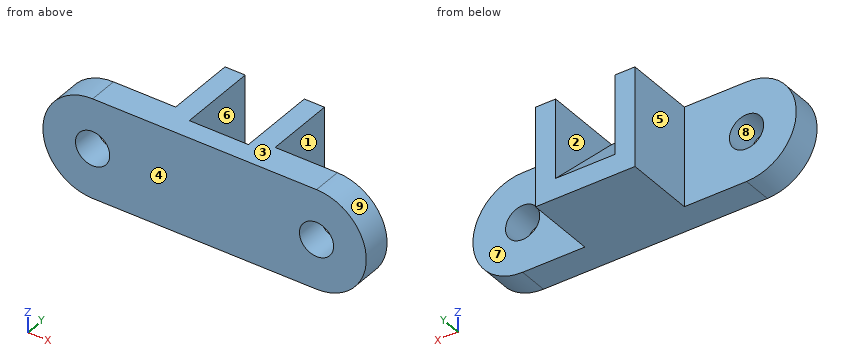
from build123d import *

# Parameters (mm, degrees)
SKETCH1_R           = 11
BOSS_EXTRUDE1_DEPTH = 19
SKETCH2_W           = 64
SKETCH2_H           = 64
BOSS_EXTRUDE2_DEPTH = 45
CUT_EXTRUDE2_START  = -13
CUT_EXTRUDE2_DEPTH  = 38


with BuildPart() as part:
    # Sketch1 → Boss-Extrude1 (new body)
    with BuildSketch(Plane(origin=(0, 0, 0), x_dir=(1, 0, 0), z_dir=(0, 1, 0))):
        with BuildLine():
            Line((-72, 32), (72, 32))
            ThreePointArc((72, 32), (104, 0), (72, -32))
            Line((72, -32), (-72, -32))
            ThreePointArc((-72, -32), (-104, 0), (-72, 32))
        make_face()
        with Locations(Location((-72, 0, 0), (0, 0, 270))):
            Circle(SKETCH1_R, mode=Mode.SUBTRACT)
        with Locations(Location((72, 0, 0), (0, 0, 270))):
            Circle(SKETCH1_R, mode=Mode.SUBTRACT)
    extrude(amount=BOSS_EXTRUDE1_DEPTH)

    # Sketch2 → Boss-Extrude2 (add)
    with BuildSketch(Plane(origin=(0, 19, 0), x_dir=(1, 0, 0), z_dir=(0, 1, 0))):
        Rectangle(SKETCH2_W, SKETCH2_H)
    extrude(amount=BOSS_EXTRUDE2_DEPTH)

    # Sketch4 → Cut-Extrude2 (cut)
    with BuildSketch(Plane.ZY.offset(32).offset(CUT_EXTRUDE2_START)):
        Polygon((32, 64), (-19, 64), (32, 13), align=None)
    extrude(amount=-CUT_EXTRUDE2_DEPTH, mode=Mode.SUBTRACT)


solid = part.part
The model under review builds one solid part; all positions refer to its coordinate system, in mm. Face numbers are marked on the shaded views. A direction names the side the tool comes from. Round coordinates to 2 decimals unless told otherwise and drop trailing zeros. Loops run counter-clockwise (first coordinate to the right, second up) from the corner with the lowest first, then second, coordinate; pieces in that order, holes last. Notation, with made-up numbers: (-39, 8) -> (-21, 8) arc R31 cw to (-21, 35) -> close; hole circle Ø3 at (-1.75, 20). An arc over 180 degrees is marked (long way). One line per question, with ' | ' between items. Start each with the question number.
Item 1: Wall thickness on line 1 along X through (y, z) = (7.75, 0); line 2 along X through (y, z) = (46, 2.5); line 3 along X through (y, z) = (7, -6.5): over which ranges is each line inside the solid? List them lowest first. Write a range as [from, to].
Item 2: Machinability: for the marked faces 1, 2, 3, 4 and 5, which of the approach directions +Z, -Z, +X, -X, +Y, -Y give a long, thin tool a straight path to every point of the face, cutting with its end or side? Answer none if there is none.
Item 3: Add section C-C, the plane x = 63.5. Write out the cut boundary in (y, z).
Item 4: For pin 1 (12 mm diameter, centred on y = 31.5, z = 15, fed in from -X); pin 2 (3 mm diameter, centred on y = 29.5, z = -7, fed in from +X); pin 3 (19 mm diameter, centred on x = 74, z = -3, fed in from +Y), all flat-tipped, find the tip position at first contact; note any pin that passes through.
Item 5: Draft analysis for pull direction X (two halves, no side actions). For the marked faces 6, 7, 8 and 9, state which applies: +X half, -X half, draft (parallel to the pull), parting line (faces both ways), or undercut.
Item 6: Add section A-A, the plane z = 0. Write out the cut boundary in (x, y).
Item 7: Add section B-B, the plane y = 57. Write out the cut boundary in (x, z), then the cut area to 3 significant figures.
Item 8: Add section D-D, the plane y = 41.5. Write out the cut boundary in (x, z), then the cut area to 3 significant figures.
Return value:
1) line 1: x = [-104, -83], [-61, 61], [83, 104] | line 2: x = [-32, -19], [19, 32] | line 3: x = [-103.33, -80.87], [-63.13, 63.13], [80.87, 103.33]
2) face 1: +Z, -Z, +X, +Y | face 2: +Z, +Y | face 3: +Z, +X, -X, +Y, -Y | face 4: +Z, -Z, +X, -X, -Y | face 5: +Z, -Z, -X, +Y
3) outline: (0, -32) -> (19, -32) -> (19, -6.98) -> (0, -6.98) -> close; (0, 6.98) -> (19, 6.98) -> (19, 32) -> (0, 32) -> close
4) pin 1: stops at x = -32 | pin 2: stops at x = 32 | pin 3: stops at y = 19
5) face 6: undercut | face 7: draft | face 8: undercut | face 9: +X half
6) outline: (-104, 0) -> (-83, 0) -> (-83, 19) -> (-104, 19) -> close; (-61, 0) -> (61, 0) -> (61, 19) -> (32, 19) -> (32, 64) -> (19, 64) -> (19, 45) -> (-19, 45) -> (-19, 64) -> (-32, 64) -> (-32, 19) -> (-61, 19) -> close; (83, 0) -> (104, 0) -> (104, 19) -> (83, 19) -> close
7) outline: (-32, -32) -> (32, -32) -> (32, 32) -> (19, 32) -> (19, -12) -> (-19, -12) -> (-19, 32) -> (-32, 32) -> close | area: 2,420 mm2
8) outline: (-32, -32) -> (32, -32) -> (32, 32) -> (19, 32) -> (19, 3.5) -> (-19, 3.5) -> (-19, 32) -> (-32, 32) -> close | area: 3,010 mm2
